Can you work these out from the model? Positions are in its coordinate system, mm. A direction names the side the tool comes from. Coordinates: 2 decimals unless noted, no trailing zeros. Order: outer loops, then holes, each group sorted by start corner. A loop starts at its lowest first (then second) coordinate and runs counter-clockwise, first axis right, second up. Notation, with made-up numbers: (24, 81.25) -> (77, 81.25) arc R19 cw to (77, 111.25) -> close; hole circle Ø9 at (41.25, 86). An arc over 180 degrees is marked (long way). Answer as a JSON object with one key per item and string values. Group by question number.
(1) I want a section at A-A, the plane z = -13.5. List the corners of the cut face in (x, y) for me, plus the area to 3 significant figures.
(2) I want a section at C-C, the plane y = 4.75. List the corners of the cut face in (x, z) for me, plus the area to 3 significant figures.
(3) I need wall thicknesses on line 1 (X direction, y = 1.2, z = -13.5); line 2 (X direction, y = 4.25, z = -13.5); line 3 (Y direction, x = -1, z = 8.5). Which ranges of each line are inside material? Lowest first, please.
(4) I want a section at B-B, the plane x = 0. List the corners of the cut face in (y, z) for me, plus the area to 3 significant figures.
(5) I want a section at D-D, the plane z = 19.5. List the corners of the cut face in (x, y) for me.
(6) Which directions (+Z, -Z, +X, -X, +Y, -Y) give clear straight access to the entire face, cutting with the end or side of a thin tool? Please do faces 1 (the flat face through (2, 8.6, -13)), 2 (the cylindrical face through (0, 6, -11)).
(7) For pin 1 (1 mm diameter, centred on x = -1, y = 5.5, fed in from +Z); pin 2 (8 mm diameter, centred on x = -2.5, z = -6.5, fed in from +Y), each with a flat end and sliding along its axis, tell me the tip position at first contact or that it passes through.
from build123d import *

# Parameters (mm, degrees)
SKETCH1_W           = 20
SKETCH1_H           = 50
BOSS_EXTRUDE1_DEPTH = 3
SKETCH3_R           = 1.6
CUT_EXTRUDE1_DEPTH  = 10
SKETCH4_R           = 2.5
SKETCH4_R_2         = 1.599999999
BOSS_EXTRUDE4_DEPTH = 5.6
FILLET1_R           = 3


with BuildPart() as part:
    # Sketch1 → Boss-Extrude1 (new body)
    with BuildSketch(Plane(origin=(0, 0, 0), x_dir=(1, 0, 0), z_dir=(0, 1, 0))):
        Rectangle(SKETCH1_W, SKETCH1_H)
    extrude(amount=BOSS_EXTRUDE1_DEPTH)

    # Sketch3 → Cut-Extrude1 (cut)
    with BuildSketch(Plane.XZ):
        with Locations(Location((0, -13.5, 0), (0, 0, 270))):
            Circle(SKETCH3_R)
    extrude(amount=-CUT_EXTRUDE1_DEPTH, mode=Mode.SUBTRACT)

    # Sketch4 → Boss-Extrude4 (add)
    with BuildSketch(Plane(origin=(0, 3, 0), x_dir=(1, 0, 0), z_dir=(0, 1, 0))):
        with Locations(Location((1e-09, 13.5, 0), (0, 0, 90))):
            Circle(SKETCH4_R)
        with Locations(Location((1e-09, 13.5, 0), (0, 0, 90.000000022))):
            Circle(SKETCH4_R_2, mode=Mode.SUBTRACT)
    extrude(amount=BOSS_EXTRUDE4_DEPTH)

    # Fillet1
    fillet1_edges = [part.edges().sort_by_distance(p)[0] for p in [
        (10, 1.5, 25),
        (-10, 1.5, 25),
    ]]
    fillet(fillet1_edges, radius=FILLET1_R)


solid = part.part
Computed values:
{
 "1": {"outline": "(-10, 0) -> (-1.6, 0) -> (-1.6, 8.6) -> (-2.5, 8.6) -> (-2.5, 3) -> (-10, 3) -> close; (1.6, 0) -> (10, 0) -> (10, 3) -> (2.5, 3) -> (2.5, 8.6) -> (1.6, 8.6) -> close", "area": "60.5 mm2"},
 "2": {"outline": "circle Ø5 at (0, -13.5); hole circle Ø3.2 at (0, -13.5)", "area": "11.6 mm2"},
 "3": {"line 1": "x = -10 to -1.6, 1.6 to 10", "line 2": "x = -2.5 to -1.6, 1.6 to 2.5", "line 3": "y = 0 to 3"},
 "4": {"outline": "(0, -25) -> (3, -25) -> (3, -16) -> (8.6, -16) -> (8.6, -15.1) -> (0, -15.1) -> close; (0, -11.9) -> (8.6, -11.9) -> (8.6, -11) -> (3, -11) -> (3, 25) -> (0, 25) -> close", "area": "150 mm2"},
 "5": {"outline": "(-10, 0) -> (10, 0) -> (10, 3) -> (-10, 3) -> close"},
 "6": {"face 1": "+Z, -Z, +X, -X, +Y", "face 2": "+Y"},
 "7": {"pin 1": "stops at z = -11.05", "pin 2": "stops at y = 3"}
}
